Solid Edge part; units mm, degrees
sketch "Sketch1" plane through (0, 0, 0) normal (0, -1, 0) x (1, 0, 0)
  circle A0 centre (0, 0) radius 4.635
extrude "Protrusion1" add sketch "Sketch1" along normal mid plane 28.38
sketch "Sketch2" plane through (0, -14.19, 0) normal (0, -1, 0) x (1, 0, 0)
  line L0 (-2.39, 3.9713) -> (-2.39, -3.9713)
  arc A0 (-2.39, -3.9713) -> (-2.39, 3.9713) centre (0, 0) cw
  line L1 (2.39, 3.9713) -> (2.39, -3.9713)
  arc A1 (2.39, -3.9713) -> (2.39, 3.9713) centre (0, 0) ccw
extrude "Enlèvement_matière_1" cut sketch "Sketch2" against normal blind 5.84
sketch "Sketch3" plane through (0, 14.19, 0) normal (0, 1, 0) x (-1, 0, 0)
  line L0 (-2.39, 3.9713) -> (-2.39, -3.9713)
  arc A0 (-2.39, -3.9713) -> (-2.39, 3.9713) centre (0, 0) cw
  line L1 (2.39, 3.9713) -> (2.39, -3.9713)
  arc A1 (2.39, 3.9713) -> (2.39, -3.9713) centre (0, 0) cw
extrude "Enlèvement_matière_2" cut sketch "Sketch3" against normal blind 6.73
Source: CAD feature listing. Evaluate the final solid. Frame: model axes, mm. A direction names the side the tool comes from. Round coordinates to 2 decimals unless told otherwise and drop trailing zeros. Loops run counter-clockwise (first coordinate to the right, second up) from the corner with the lowest first, then second, coordinate; pieces in that order, holes last. Notation, with made-up numbers: M -23,56 L 31,56 A31 cw 31,92 Z; hole C -27,-33.75 d1. An arc over 180 degrees is marked long. Put each result on its own line as item: value.
(1) Section B-B, the plane y = -9.25. Return loops of the section in (x, z) (3 decimals), and give its area (3 significant figures).
Solutions:
outline: M -2.39,-3.971 A4.635 ccw 2.39,-3.971 L 2.39,3.971 A4.635 ccw -2.39,3.971 Z
area: 42.3 mm²
(2) Section C-C, the plane x = -1.75. Return loops of the section in (y, z).
Solutions:
outline: M -14.19,-4.29 L 14.19,-4.29 L 14.19,4.29 L -14.19,4.29 Z
(3) Pull-direction query (Z, two-part tool) for faces 5 (the face through (2.14, 0.2, 4.11)), 6 (the face through (3, 7.46, 0)); classes: released by +Z, released by -Z, zero draft, split by the parting line, or undercut.
Solutions:
face 5: split by the parting line
face 6: zero draft
(4) Ray query, line 1 (X direction, y = 7.5, z = 2.5); line 2 (Y direction, x = 2.5, z = 2.75); line 3 (X direction, y = 5.5, z = -1.25). Return the intervals inside material, ascending. Write a range as [from, to].
Solutions:
line 1: [-2.39, 2.39]
line 2: [-8.35, 7.46]
line 3: [-4.46, 4.46]
(5) Access query for faces 1 (the face through (-3, 7.46, 0)), 2 (the face through (-2.39, -11, 0)), 3 (the face through (3, -8.35, 0)), 4 (the face through (2.39, 11, 0)). Directions: +Z, -Z, +X, -X, +Y, -Y. A direction counts if a zero-diameter tool reaches every point of the face in a straight line with its end or side. Return the directions, or none.
Solutions:
face 1: +Z, -Z, -X, +Y
face 2: +Z, -Z, -X, -Y
face 3: +Z, -Z, +X, -Y
face 4: +Z, -Z, +X, +Y
(6) First-contact query: pin 1 (1.1 mm diameter, centred on x = 3, z = -0.5, fed in from -Y); pin 2 (1.5 mm diameter, centred on y = 9.5, z = 3.5, fed in from +X); pin 3 (3 mm diameter, centred on x = 3.5, y = 10, fed in from -Z); pin 4 (4 mm diameter, centred on y = -9, z = -2, fed in from +X). Flat tips, straight axial feed; report the tip coordinate or a pass-through.
Solutions:
pin 1: y = -8.35
pin 2: x = 2.39
pin 3: z = -4.18
pin 4: x = 4.63
(7) Section A-A, the plane z = 0. Return loops of the section in (x, y) (3 decimals), and give its area (3 significant figures).
Solutions:
outline: M -4.635,-8.35 L -2.39,-8.35 L -2.39,-14.19 L 2.39,-14.19 L 2.39,-8.35 L 4.635,-8.35 L 4.635,7.46 L 2.39,7.46 L 2.39,14.19 L -2.39,14.19 L -2.39,7.46 L -4.635,7.46 Z
area: 207 mm²
(8) Section D-D, the plane z = -1.75. Return loops of the section in (x, y).
Solutions:
outline: M -4.29,-8.35 L -2.39,-8.35 L -2.39,-14.19 L 2.39,-14.19 L 2.39,-8.35 L 4.29,-8.35 L 4.29,7.46 L 2.39,7.46 L 2.39,14.19 L -2.39,14.19 L -2.39,7.46 L -4.29,7.46 Z
